The listing builds one solid part. Answer for the finished solid, in the listing's coordinates (mm). Round coordinates to 2 decimals unless told otherwise and drop trailing zeros. Order: outer loops, then holes, each group sorted by start corner. A loop starts at its lowest first (then second) coordinate and runs counter-clockwise, first axis right, second up. Notation, with made-up numbers: (1.5, -29) - (13.5, -29) arc R18 ccw to (13.5, -19) - close; hole circle Ø11 at (-31.5, 7). An arc over 180 degrees is marked (long way). One line per item, written item: value. Start each with the question number.
1. Section A-A, the plane y = 44.45 is taken. Give the vertices of the cut face in (x, z).
2. Section B-B, the plane z = 4.5 is taken. Give the vertices of the cut face in (x, y), then the cut area to 3 significant figures.
3. Section C-C, the plane x = 2.7 is taken. Give the vertices of the cut face in (y, z).
4. For a pull along X with two mould halves and no side action, classify faces 1 (the flat face through (5.08, 31, 4)), 2 (the flat face through (3, 63.5, 4)), 3 (the flat face through (0, 31, 4)) as released by +X, released by -X, zero draft, split by the parting line, or undercut.
5. Flat-ended cylindrical pins translate along their axes: P1, Ø2.5, axis at y = 44.45, z = 3.74, coming from the +X side; P2, Ø2, axis at y = 30.5, z = 3, coming from the -X side. Find the tip coordinate at first contact, or state that the pin passes through.
6. Straight lines are drawn through the part: line 1 (Y direction, x = 4.1, z = 4.5); line 2 (Y direction, x = 2.7, z = 4.25); line 3 (Z direction, x = 3.75, y = 43.5). For each, find the intervals that lie inside material, in ascending order.
from build123d import *

# Parameters (mm, degrees)
SKETCH1_W           = 5.08
SKETCH1_H           = 63.5
BOSS_EXTRUDE1_DEPTH = 7.62
SKETCH2_R           = 1.5
CUT_EXTRUDE1_DEPTH  = 6.08


with BuildPart() as part:
    # Sketch1 → Boss-Extrude1 (new body)
    with BuildSketch(Plane.XY):
        with Locations((2.54, 31.75)):
            Rectangle(SKETCH1_W, SKETCH1_H)
    extrude(amount=BOSS_EXTRUDE1_DEPTH)

    # Sketch2 → Cut-Extrude1 (cut, through all)
    with BuildSketch(Plane.ZY):
        with Locations((3.744499847, 57.658)):
            Circle(SKETCH2_R)
        with Locations((3.744499847, 44.45)):
            Circle(SKETCH2_R)
    extrude(amount=-CUT_EXTRUDE1_DEPTH, mode=Mode.SUBTRACT)


solid = part.part
Answer list:
1. outline: (0, 0) - (5.08, 0) - (5.08, 2.24) - (0, 2.24) - close; (0, 5.24) - (5.08, 5.24) - (5.08, 7.62) - (0, 7.62) - close
2. outline: (0, 0) - (5.08, 0) - (5.08, 43.15) - (0, 43.15) - close; (0, 45.75) - (5.08, 45.75) - (5.08, 56.36) - (0, 56.36) - close; (0, 58.95) - (5.08, 58.95) - (5.08, 63.5) - (0, 63.5) - close
2. area: 296 mm²
3. outline: (0, 0) - (63.5, 0) - (63.5, 7.62) - (0, 7.62) - close; hole circle Ø3 at (44.45, 3.74); hole circle Ø3 at (57.66, 3.74)
4. face 1: released by +X
4. face 2: zero draft
4. face 3: released by -X
5. P1: passes through
5. P2: stops at x = 0
6. line 1: y = 0 to 43.15, 45.75 to 56.36, 58.95 to 63.5
6. line 2: y = 0 to 43.04, 45.86 to 56.25, 59.07 to 63.5
6. line 3: z = 0 to 2.58, 4.91 to 7.62
